Source: three-view drawing plus pictorial views. Frame: mm from the lowest corner of the part. A direction names the side the tool comes from. Round coordinates to 2 decimals unless told otherwise and drop trailing zeros. Loops run counter-clockwise (first coordinate to the right, second up) from the corner with the lowest first, then second, coordinate; pieces in that order, holes last. Notation, with made-up numbers: M 14,-25 L 48,-25 A30 ccw 48,5 Z; hole C 49.25,83 d3. An arc over 180 degrees is marked long. Answer as a JSON object with one key per item and string values.
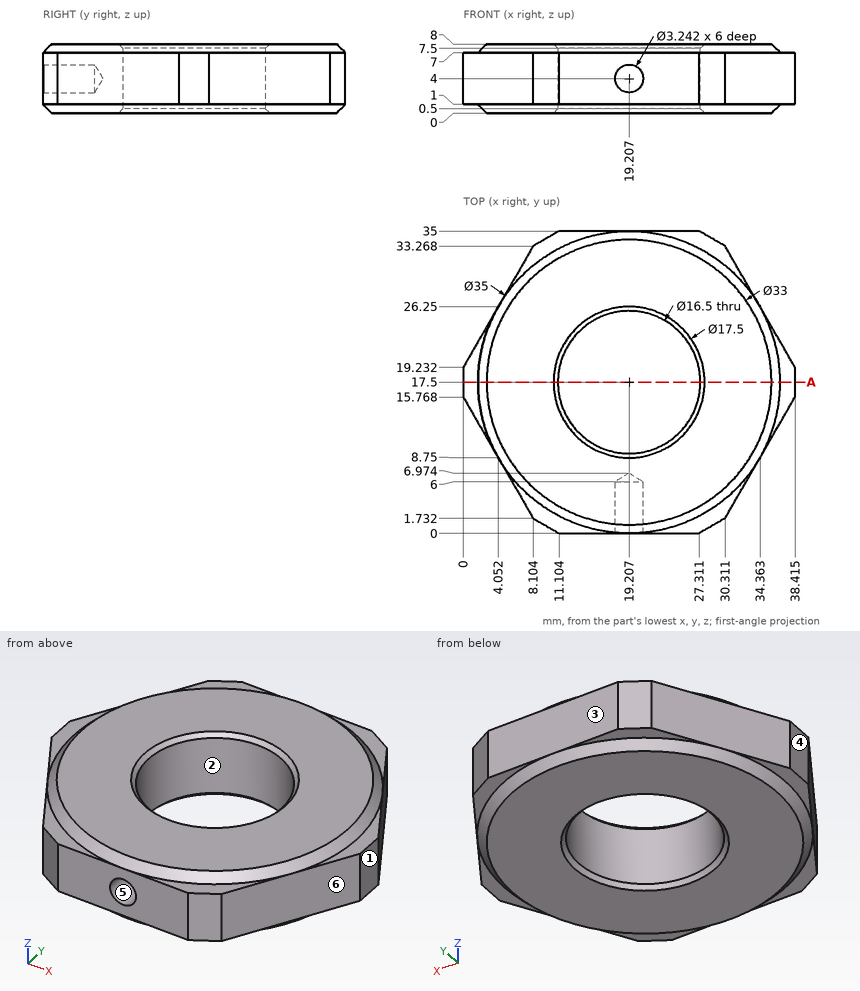
1) Cut plane A-A on y = 17.5. Return the cut outline in (x, z) (1 decimal).
Geometry results:
{"outline": "M 0,1 L 1.7,1 L 2.7,0 L 10.5,0 L 11,0.5 L 11,7.5 L 10.5,8 L 2.7,8 L 1.7,7 L 0,7 Z; M 27.5,0.5 L 28,0 L 35.7,0 L 36.7,1 L 38.4,1 L 38.4,7 L 36.7,7 L 35.7,8 L 28,8 L 27.5,7.5 Z"}
2) Pull-direction query (X, two-part tool) for the marked faces 1, 2, 3 and 4; classes: +X half, -X half, draft (parallel to the pull), parting line (faces both ways), or undercut.
Geometry results:
{"face 1": "+X half", "face 2": "undercut", "face 3": "draft", "face 4": "-X half"}
3) Line query: probe 1 along Y at (x, z) = (19, 6); probe 2 along Y at (x, z) = (26, 1.5) (1 decimal); probe 3 along X at (y, z) = (3.5, 2.75) (1 decimal). Output: solid intervals per line, ascending.
Geometry results:
{"probe 1": "0 to 9.25, 25.75 to 35", "probe 2": "0 to 12.8, 22.2 to 35", "probe 3": "7.1 to 18.2, 20.2 to 31.3"}
4) Set-up query: the marked faces 5 and 6. Return all of +Z, -Z, +X, -X, +Y, -Y with unobstructed straight access to the full face (end or side cutting, diameter ignored); none if empty.
Geometry results:
{"face 5": "-Y", "face 6": "+Z, -Z, +X, -Y"}
5) First-contact query: pin 1 (8 mm diameter, centred on x = 29.5, y = 4, fed in from +Z); pin 2 (1.2 mm diameter, centred on x = 1.5, y = 19.5, fed in from -Z); pin 3 (2 mm diameter, centred on x = 13.5, y = 19.5, fed in from +Z); pin 4 (3 mm diameter, centred on x = 8.5, z = 7, fed in from +Y). Flat tips, straight axial feed; report the tip coordinate or a pass-through.
Geometry results:
{"pin 1": "z = 8", "pin 2": "z = 0.72", "pin 3": "through", "pin 4": "y = 34.36"}
